The listing builds one solid part. Answer for the finished solid, in the listing's coordinates (mm). A direction names the side the tool comes from. Coordinates: 2 decimals unless noted, no trailing zeros. Order: outer loops, then holes, each group sorted by start corner. A loop starts at its lowest first (then second) coordinate and runs counter-clockwise, first axis right, second up. Notation, with made-up numbers: (-22.5, 68) -> (7.5, 68) arc R20 cw to (7.5, 97) -> close; hole circle Ø5 at (-26, 64). An arc over 180 degrees is marked (long way). Write item = value, one per line.
from build123d import *

# Parameters (mm, degrees)
SKETCH1_R               = 5
BOSS_EXTRUDE1_DEPTH     = 104.75
SKETCH5_R               = 5
SKETCH5_R_2             = 3.975
CUT_EXTRUDE3_DEPTH      = 199.15
CUT_EXTRUDE4_DEPTH      = 2
CUT_EXTRUDE5_DEPTH      = 2
SKETCH11_R              = 1.3
CUT_EXTRUDE6_DEPTH      = 1
CUT_EXTRUDE7_START      = -1
SKETCH12_R              = 1.3
CUT_EXTRUDE7_DEPTH      = 1
CUT_EXTRUDE8_DEPTH      = 105.988392216
CUT_EXTRUDE8_DEPTH_BACK = 105.988392216
SKETCH13_R              = 1.065


with BuildPart() as part:
    # Sketch1 → Boss-Extrude1 (new, symmetric)
    with BuildSketch(Plane(origin=(0, 0, 0), x_dir=(1, 0, 0), z_dir=(0, 1, 0))):
        with Locations(Location((0, 0, 0), (0, 0, 270))):
            Circle(SKETCH1_R)
    extrude(amount=BOSS_EXTRUDE1_DEPTH, both=True)

    # Sketch5 → Cut-Extrude3 (cut)
    with BuildSketch(Plane(origin=(0, 104.75, 0), x_dir=(1, 0, 0), z_dir=(0, 1, 0))):
        with Locations(Location((0, 0, 0), (0, 0, 270))):
            Circle(SKETCH5_R)
        with Locations(Location((0, 0, 0), (0, 0, 270))):
            Circle(SKETCH5_R_2, mode=Mode.SUBTRACT)
    extrude(amount=-CUT_EXTRUDE3_DEPTH, mode=Mode.SUBTRACT)

    # Sketch8 → Cut-Extrude4 (cut)
    with BuildSketch(Plane(origin=(0, 104.75, 0), x_dir=(1, 0, 0), z_dir=(0, 1, 0))):
        Polygon((1.173959492, 2.088696351), (-1.221884355, 2.061026918), (-2.395843846, -0.027669433), (-1.173959492, -2.088696351), (1.221884355, -2.061026918), (2.395843846, 0.027669433), align=None)
    extrude(amount=-CUT_EXTRUDE4_DEPTH, mode=Mode.SUBTRACT)

    # Sketch10 → Cut-Extrude5 (cut)
    with BuildSketch(Plane.XZ.offset(104.75)):
        Polygon((0, 2.396003617), (-2.075, 1.198001809), (-2.075, -1.198001809), (0, -2.396003617), (2.075, -1.198001809), (2.075, 1.198001809), align=None)
    extrude(amount=-CUT_EXTRUDE5_DEPTH, mode=Mode.SUBTRACT)

    # Sketch11 → Cut-Extrude6 (cut)
    with BuildSketch(Plane.XZ.offset(102.75)):
        with Locations(Location((0, 0, 0), (0, 0, 270))):
            Circle(SKETCH11_R)
    extrude(amount=-CUT_EXTRUDE6_DEPTH, mode=Mode.SUBTRACT)

    # Sketch12 → Cut-Extrude7 (cut)
    with BuildSketch(Plane(origin=(0, 102.75, 0), x_dir=(1, 0, 0), z_dir=(0, 1, 0)).offset(CUT_EXTRUDE7_START)):
        with Locations(Location((0, 0, 0), (0, 0, 90))):
            Circle(SKETCH12_R)
    extrude(amount=CUT_EXTRUDE7_DEPTH, mode=Mode.SUBTRACT)

    # Sketch13 → Cut-Extrude8 (cut, two sides: drawn at the far end of the back side and taken through both)
    with BuildSketch(Plane(origin=(0, 0, 0), x_dir=(0, 0, -1), z_dir=(1, 0, 0)).offset(-CUT_EXTRUDE8_DEPTH_BACK)):
        with Locations(Location((-0.027669433, 98.55, 0), (0, 0, 180))):
            Circle(SKETCH13_R)
    extrude(amount=CUT_EXTRUDE8_DEPTH + CUT_EXTRUDE8_DEPTH_BACK, mode=Mode.SUBTRACT)


solid = part.part
Q1. Find the intervals of material crossed by line 1 along X through (y, z) = (-102.35, 0); line 2 along Y through (x, z) = (-2, 0.25); line 3 along Z through (x, y) = (0.25, 98.55), in increasing order.
The answers:
line_1 = -5 to -1.3, 1.3 to 5
line_2 = -102.75 to 97.51, 99.59 to 102.75
line_3 = -3.97 to -1.04, 1.09 to 3.97
Q2. Section A-A, the plane y = 24.5 is taken. Give the vertices of the cut face in (x, z) (3 decimals), plus the area to 3 significant figures.
The answers:
outline = circle Ø7.95 at (0, 0)
area = 49.6 mm2
Q3. The mould has two halves that part along X. Classify faces 1 (the face through (2, 102.75, 0)), 2 (the face through (-2.419, 6.569, -3.154)), 3 (the face through (-2, 104.75, 2)), 4 (the face through (0, -102.75, -2)): released by +X, released by -X, zero draft, split by the parting line, or undercut.
The answers:
face_1 = undercut
face_2 = split by the parting line
face_3 = zero draft
face_4 = undercut
Q4. A tool of negligible diameter and unlimited length cuts with its end or side. For faces 5 (the face through (-4.88, -99.5, -1.08)), 6 (the face through (-4, -94.4, -2)), from which of +Z, -Z, +X, -X, +Y, -Y can it reach the whole face along a straight path? Write none if from no direction.
The answers:
face_5 = +Y, -Y
face_6 = +Y
Q5. Each of these flat-tipped pins is pushed along its axis until it touches: pin 1 Ø2 at (x, z) = (0, 0.5) entering from +Y; pin 2 Ø2 at (x, y) = (-0.5, -11) entering from +Z (3 decimals); pin 3 Ø2 at (x, z) = (0.5, 0.5) entering from -Y. Where does it stop, or does it pass through?
The answers:
pin_1 = 102.75
pin_2 = 3.975
pin_3 = -102.75
